Source: CAD feature listing. Evaluate the final solid. Frame: model axes, mm. A direction names the side the tool comes from. Round coordinates to 2 decimals unless told otherwise and drop trailing zeros. Order: outer loops, then holes, each group sorted by start corner. A loop starts at its lowest first (then second) coordinate and runs counter-clockwise, first axis right, second up.
```python
from build123d import *

# Parameters (mm, degrees)
SKETCH1_W           = 10
SKETCH1_H           = 5
SKETCH1_H_2         = 10
SKETCH1_W_2         = 5
BOSS_EXTRUDE1_DEPTH = 5
SKETCH2_R           = 2.8067
CUT_EXTRUDE1_DEPTH  = 5
CIRPATTERN1_COUNT   = 4


with BuildPart() as part:
    # Sketch1 → Boss-Extrude1 (new, symmetric)
    with BuildSketch(Plane(origin=(0, 0, 0), x_dir=(1, 0, 0), z_dir=(0, 1, 0))):
        with Locations((0, -7.5)):
            Rectangle(SKETCH1_W, SKETCH1_H)
        Rectangle(SKETCH1_W, SKETCH1_H_2)
        with Locations((-7.5, 0)):
            Rectangle(SKETCH1_W_2, SKETCH1_H_2)
        with Locations((7.5, 0)):
            Rectangle(SKETCH1_W_2, SKETCH1_H_2)
        with Locations((0, 7.5)):
            Rectangle(SKETCH1_W, SKETCH1_H)
    extrude(amount=BOSS_EXTRUDE1_DEPTH, both=True)

    # Sketch2 → Cut-Extrude1 (cut)
    with BuildSketch(Plane.XY.offset(10)):
        Circle(SKETCH2_R)
    cut_extrude1 = extrude(amount=-CUT_EXTRUDE1_DEPTH, mode=Mode.SUBTRACT)

    # CirPattern1: Cut-Extrude1 ×4 about axis
    cirpattern1_axis = Axis((0, 0, 0), (0, 1, 0))
    for i in range(1, CIRPATTERN1_COUNT):
        add(cut_extrude1.rotate(cirpattern1_axis, i * 360 / CIRPATTERN1_COUNT), mode=Mode.SUBTRACT)


solid = part.part
```
1. Section D-D on x = 0. Return loops of the section in (y, z), plus the area to 3 significant figures.
2. First-contact query: pin 1 (4 mm diameter, centred on x = 7.5, y = -2, fed in from +Z); pin 2 (2.5 mm diameter, centred on y = 2.5, z = 7.5, fed in from +X); pin 3 (4 mm diameter, centred on y = 0.5, z = -7.5, fed in from -X). Flat tips, straight axial feed; report the tip coordinate or a pass-through.
3. Access query for faces 1 (the face through (-7.54, 0.84, 2.68)), 2 (the face through (5, 0, -7)), 3 (the face through (0.61, -2.74, -7.54)), 4 (the face through (7.54, 0.84, -2.68)). Directions: +Z, -Z, +X, -X, +Y, -Y. A direction counts if a zero-diameter tool reaches every point of the face in a straight line with its end or side. Return the directions, or none.
4. Section A-A on z = 7. Return loops of the section in (x, y).
5. Pull-direction query (X, two-part tool) for faces 5 (the face through (-5, 0, 7)), 6 (the face through (0, 0, 5)), 7 (the face through (0, 5, 0)), 8 (the face through (10, 2.3, -2.2)); classes: released by +X, released by -X, zero draft, split by the parting line, or undercut.
6. Section C-C on y = 0. Return loops of the section in (x, z), plus the area to 3 significant figures.
7. Line query: line 1 along Y through (x, z) = (0, 7.75); line 2 along Z through (x, y) = (-5.5, 4.75); line 3 along Z through (x, y) = (7.25, -2.5). Output: solid intervals per line, ascending.
Result:
1. outline: (-5, -10) - (-2.81, -10) - (-2.81, -5) - (2.81, -5) - (2.81, -10) - (5, -10) - (5, 10) - (2.81, 10) - (2.81, 5) - (-2.81, 5) - (-2.81, 10) - (-5, 10) - close
1. area: 144 mm2
2. pin 1: stops at z = 5
2. pin 2: stops at x = 5
2. pin 3: stops at x = -5
3. face 1: -X
3. face 2: -Z, +X, +Y, -Y
3. face 3: -Z
3. face 4: +X
4. outline: (-5, -5) - (5, -5) - (5, 5) - (-5, 5) - close; hole circle Ø5.61 at (0, 0)
5. face 5: released by -X
5. face 6: undercut
5. face 7: zero draft
5. face 8: released by +X
6. outline: (-10, -5) - (-5, -5) - (-5, -10) - (-2.81, -10) - (-2.81, -5) - (2.81, -5) - (2.81, -10) - (5, -10) - (5, -5) - (10, -5) - (10, -2.81) - (5, -2.81) - (5, 2.81) - (10, 2.81) - (10, 5) - (5, 5) - (5, 10) - (2.81, 10) - (2.81, 5) - (-2.81, 5) - (-2.81, 10) - (-5, 10) - (-5, 5) - (-10, 5) - (-10, 2.81) - (-5, 2.81) - (-5, -2.81) - (-10, -2.81) - close
6. area: 188 mm2
7. line 1: y = -5 to -2.81, 2.81 to 5
7. line 2: z = -5 to 5
7. line 3: z = -5 to -1.28, 1.28 to 5
